Check sheet for the modelled part. Datum: model origin and axes. Units: mm. A direction names the side the tool comes from. Give positions to 0.01 mm unless a question says otherwise; leave off trailing zeros. Loops run counter-clockwise (first coordinate to the right, second up) from the corner with the lowest first, then second, coordinate; pieces in that order, holes last. Notation, with made-up numbers: (84.25, 44.5) -> (120.25, 44.5) arc R21 ccw to (120.25, 77.5) -> close; hole circle Ø5 at (80, 69). An arc over 180 degrees is marked (long way). Write each question's results on one line, items separated by ' | '. Start each with the question number.
Item 1: Cross-section at C-C on y = 28. Enter the section's corners in (x, z).
Item 2: Cross-section at A-A on z = 0. Enter the section's corners in (x, y).
Item 3: Cross-section at D-D on z = 2. Enter the section's corners in (x, y), then the cut area to 3 significant figures.
Item 4: Scan lines: line 1 along Y through (x, z) = (5.25, -2.5); line 2 along Z through (x, y) = (0.25, 15); line 3 along X through (y, z) = (21, -1.75). Record each from-to range of solid material in increasing order.
Item 5: Cross-section at B-B on x = -4.25. Enter the section's corners in (y, z).
Item 6: Gauge pin test, flat ends, axial feed: pin 1 Ø2 at (x, y) = (-0.5, 12) entering from -Z; pin 2 Ø5 at (x, y) = (-3.5, 13) entering from -Z; pin 3 Ø3 at (y, z) = (21.5, -3.5) entering from +X. Record the tip position at first contact, or that the pin passes through.
Item 7: Access from +Z, -Z, +X, -X, +Y, -Y to the whole of each face (thin tool, end or side, straight path). Record for faces 1 (the face through (1.5, 31.97, -0.07)), 2 (the face through (0.794, 9.86, -6.044)), 3 (the face through (0, 0, 0)).
Autodesk Inventor part; units mm, degrees
ref_plane "YZ Plane" through (0, 0, 0) normal (1, 0, 0) x (0, 1, 0)
ref_plane "XZ Plane" through (0, 0, 0) normal (0, 1, 0) x (-1, 0, 0)
ref_plane "XY Plane" through (0, 0, 0) normal (0, 0, 1) x (1, 0, 0)
sketch "Sketch1" plane through (0, 0, 0) normal (0, 0, 1) x (1, 0, 0)
  line L0 (0, 34) -> (-1.5, 34)
  line L1 (-1.5, 34) -> (-1.5, 30)
  line L2 (-1.5, 30) -> (-6.35, 30)
  line L3 (-6.35, 30) -> (-6.35, 20)
  line L4 (-6.35, 20) -> (-6.096, 20)
  line L5 (-6.096, 20) -> (-6.096, 0)
  line L6 (-6.096, 0) -> (0, 0)
  line L7 (0, 0) -> (0, 34)
  dimension "d0" = 1.5
  dimension "d2" = 6.096
  dimension "d3" = 20
  dimension "d4" = 4
  dimension "d5" = 10
  dimension "d9" = 6.35
revolve "Revolution1" add sketch "Sketch1" angle 360 about axis through (0, 0, 0) along (0, 1, 0)
thread "Thread1"
equation "\"d2\" = 0.5 * tube_od - tube_wall"
equation "\"d9\" = 0.5 * tube_od"
properties part number "tubeFitting" material "Brass, Soft Yellow"
Answer sheet:
1) outline: circle Ø12.7 at (0, 0)
2) outline: (-6.35, 20) -> (-6.1, 20) -> (-6.1, 0) -> (6.1, 0) -> (6.1, 20) -> (6.35, 20) -> (6.35, 30) -> (1.5, 30) -> (1.5, 34) -> (-1.5, 34) -> (-1.5, 30) -> (-6.35, 30) -> close
3) outline: (-6.03, 20) -> (-5.76, 20) -> (-5.76, 0) -> (5.76, 0) -> (5.76, 20) -> (6.03, 20) -> (6.03, 30) -> (-6.03, 30) -> close | area: 351 mm²
4) line 1: y = 0 to 30 | line 2: z = -6.09 to 6.09 | line 3: x = -6.1 to 6.1
5) outline: (0, -4.37) -> (20, -4.37) -> (20, -4.72) -> (30, -4.72) -> (30, 4.72) -> (20, 4.72) -> (20, 4.37) -> (0, 4.37) -> close
6) pin 1: stops at z = -6.1 | pin 2: stops at z = -6.01 | pin 3: stops at x = 6.03
7) face 1: +Y | face 2: -Y | face 3: +Z, -Z, +X, -X, -Y
